Can you work these out from the model? Positions are in its coordinate system, mm. Give positions to 0.01 mm unless a question says otherwise; leave off trailing zeros. Loops run counter-clockwise (first coordinate to the right, second up) from the corner with the lowest first, then second, coordinate; pieces in that order, holes last. Notation, with made-up numbers: M -14.5,19.5 L 42.5,19.5 A16 ccw 42.5,39.5 Z; hole C 36,-27.5 d2. An arc over 180 degrees is marked long. Put each result on its own line as item: value. Start each with the question number.
1) Imagine slicing it at A-A (y = 88.9). Write out the boundary of the cut face in (x, z).
2) If we mould it in two halves opening along Z, with no side actions, what happens to faces 1 (the cylindrical face through (43.83, 61.02, 18.5)), 2 (the flat face through (44, 125, 38.1)), 3 (the flat face through (44, 254, 19)), 4 (the cylindrical face through (43.83, 116.82, 18.72))? For each: +Z half, -Z half, draft (parallel to the pull), parting line (faces both ways), or undercut.
3) Imagine slicing it at B-B (x = 11). State how many separate pieces and enclosed holes the cut face has, then the cut area to 3 significant figures.
from build123d import *

# Parameters (mm, degrees)
SKETCH1_W           = 88.9
SKETCH1_H           = 38.1
BOSS_EXTRUDE1_DEPTH = 254
SKETCH2_R           = 2.54
CUT_EXTRUDE1_DEPTH  = 272.7918689


with BuildPart() as part:
    # Sketch1 → Boss-Extrude1 (new body)
    with BuildSketch(Plane(origin=(0, 0, 0), x_dir=(1, 0, 0), z_dir=(0, 1, 0))):
        with Locations((44.45, -19.05)):
            Rectangle(SKETCH1_W, SKETCH1_H)
    extrude(amount=BOSS_EXTRUDE1_DEPTH)

    # Sketch2 → Cut-Extrude1 (cut, through all)
    with BuildSketch(Plane.ZY):
        with Locations((19.05, 12.7)):
            Circle(SKETCH2_R)
        with Locations((19.05, 38.1)):
            Circle(SKETCH2_R)
        with Locations((19.05, 63.5)):
            Circle(SKETCH2_R)
        with Locations((19.05, 88.9)):
            Circle(SKETCH2_R)
        with Locations((19.05, 114.3)):
            Circle(SKETCH2_R)
        with Locations((19.05, 139.7)):
            Circle(SKETCH2_R)
        with Locations((19.05, 165.1)):
            Circle(SKETCH2_R)
        with Locations((19.05, 190.5)):
            Circle(SKETCH2_R)
        with Locations((19.05, 215.9)):
            Circle(SKETCH2_R)
        with Locations((19.05, 241.3)):
            Circle(SKETCH2_R)
    extrude(amount=-CUT_EXTRUDE1_DEPTH, mode=Mode.SUBTRACT)


solid = part.part
Recorded:
1. outline: M 0,0 L 88.9,0 L 88.9,16.51 L 0,16.51 Z; M 0,21.59 L 88.9,21.59 L 88.9,38.1 L 0,38.1 Z
2. face 1: undercut
2. face 2: +Z half
2. face 3: draft
2. face 4: undercut
3. separate pieces: 1
3. enclosed holes: 10
3. area: 9,470 mm²
